Can you work these out from the model? Positions are in its coordinate system, mm. A direction names the side the tool comes from. Round coordinates to 2 decimals unless told otherwise and drop trailing zeros. Write each loop counter-clockwise with the first axis right and the second up, starting at its lowest first coordinate (ties: lowest second). Pieces come first, ordered by that corner, then holes. Notation, with made-up numbers: M -30,-7.75 L 16,-7.75 A36 ccw 16,29.25 Z; hole C -26,5.25 d10. An arc over 180 degrees is marked long. Use one line per item in the form item = value. Start each with the question number.
```python
from build123d import *

# Parameters (mm, degrees)
SKETCH1_R           = 113.19870133
BOSS_EXTRUDE1_DEPTH = 10
SKETCH3_R           = 10
BOSS_EXTRUDE2_DEPTH = 92
BOSS_EXTRUDE3_START = -10
SKETCH4_R           = 118.19870133
SKETCH4_R_2         = 113.19870133
BOSS_EXTRUDE3_DEPTH = 102
CUT_EXTRUDE1_START  = -59
CUT_EXTRUDE1_DEPTH  = 59


with BuildPart() as part:
    # Sketch1 → Boss-Extrude1 (new body)
    with BuildSketch(Plane(origin=(0, 0, 0), x_dir=(1, 0, 0), z_dir=(0, 1, 0))):
        with Locations(Location((0, 0, 0), (0, 0, 270))):
            Circle(SKETCH1_R)
    extrude(amount=BOSS_EXTRUDE1_DEPTH)

    # Sketch3 → Boss-Extrude2 (add)
    with BuildSketch(Plane(origin=(0, 10, 0), x_dir=(1, 0, 0), z_dir=(0, 1, 0))):
        with BuildLine():
            Line((11.81310243, 2.10964712), (146.802984355, 2.10964712))
            ThreePointArc((146.802984355, 2.10964712), (146.818142021, 0), (146.802984355, -2.10964712))
            Line((146.802984355, -2.10964712), (11.81310243, -2.10964712))
            ThreePointArc((11.81310243, -2.10964712), (10.811626415, -5.206604869), (9.014737429, -7.920511921))
            Line((9.014737429, -7.920511921), (93.179552163, -113.459851424))
            ThreePointArc((93.179552163, -113.459851424), (91.539614278, -114.78704563), (89.880775093, -116.090538354))
            Line((89.880775093, -116.090538354), (5.715960358, -10.55119885))
            ThreePointArc((5.715960358, -10.55119885), (2.670251207, -11.699134946), (-0.571908724, -11.986363936))
            Line((-0.571908724, -11.986363936), (-30.609983324, -143.591767687))
            ThreePointArc((-30.609983324, -143.591767687), (-32.670110084, -143.137104671), (-34.723491048, -142.652886392))
            Line((-34.723491048, -142.652886392), (-4.685416448, -11.047482641))
            ThreePointArc((-4.685416448, -11.047482641), (-7.481877622, -9.38197779), (-9.727895943, -7.02623943))
            Line((-9.727895943, -7.02623943), (-131.349577039, -65.596154143))
            ThreePointArc((-131.349577039, -65.596154143), (-132.278575204, -63.70200443), (-133.1802602, -61.794701388))
            Line((-133.1802602, -61.794701388), (-11.558579104, -3.224786676))
            ThreePointArc((-11.558579104, -3.224786676), (-12, 0), (-11.558579104, 3.224786676))
            Line((-11.558579104, 3.224786676), (-133.1802602, 61.794701388))
            ThreePointArc((-133.1802602, 61.794701388), (-132.278575204, 63.70200443), (-131.349577039, 65.596154143))
            Line((-131.349577039, 65.596154143), (-9.727895943, 7.02623943))
            ThreePointArc((-9.727895943, 7.02623943), (-7.481877622, 9.38197779), (-4.685416448, 11.047482641))
            Line((-4.685416448, 11.047482641), (-34.723491048, 142.652886392))
            ThreePointArc((-34.723491048, 142.652886392), (-32.670110084, 143.137104671), (-30.609983324, 143.591767687))
            Line((-30.609983324, 143.591767687), (-0.571908724, 11.986363936))
            ThreePointArc((-0.571908724, 11.986363936), (2.670251207, 11.699134946), (5.715960358, 10.55119885))
            Line((5.715960358, 10.55119885), (89.880775093, 116.090538354))
            ThreePointArc((89.880775093, 116.090538354), (91.539614278, 114.78704563), (93.179552163, 113.459851424))
            Line((93.179552163, 113.459851424), (9.014737429, 7.920511921))
            ThreePointArc((9.014737429, 7.920511921), (10.811626415, 5.206604869), (11.81310243, 2.10964712))
        make_face()
        with Locations(Location((0, 0, 0), (0, 0, 270))):
            Circle(SKETCH3_R, mode=Mode.SUBTRACT)
    extrude(amount=BOSS_EXTRUDE2_DEPTH)

    # Sketch4 → Boss-Extrude3 (add)
    with BuildSketch(Plane(origin=(0, 10, 0), x_dir=(1, 0, 0), z_dir=(0, 1, 0)).offset(BOSS_EXTRUDE3_START)):
        with Locations(Location((0, 0, 0), (0, 0, 270))):
            Circle(SKETCH4_R)
        Circle(SKETCH4_R_2, mode=Mode.SUBTRACT)
    extrude(amount=BOSS_EXTRUDE3_DEPTH)

    # Sketch5 → Cut-Extrude1 (cut)
    with BuildSketch(Plane(origin=(0, 10, 0), x_dir=(1, 0, 0), z_dir=(0, 1, 0)).offset(CUT_EXTRUDE1_START)):
        with BuildLine():
            Line((-113.173392965, 2.393555442), (-11.53804838, 2.393555442))
            ThreePointArc((-11.53804838, 2.393555442), (-10.204986578, 5.891851748), (-7.841904008, 8.795465286))
            Line((-7.841904008, 8.795465286), (-58.6595763, 96.814255619))
            ThreePointArc((-58.6595763, 96.814255619), (-98.032951027, 56.599350665), (-113.173392965, 2.393555442))
        make_face()
        with BuildLine():
            Line((-54.513816664, 99.207811061), (-3.696144372, 11.189020728))
            ThreePointArc((-3.696144372, 11.189020728), (0, 11.783703496), (3.696144372, 11.189020728))
            Line((3.696144372, 11.189020728), (54.513816664, 99.207811061))
            ThreePointArc((54.513816664, 99.207811061), (0, 113.19870133), (-54.513816664, 99.207811061))
        make_face()
        with BuildLine():
            Line((-58.6595763, -96.814255619), (-7.841904008, -8.795465286))
            ThreePointArc((-7.841904008, -8.795465286), (-10.204986578, -5.891851748), (-11.53804838, -2.393555442))
            Line((-11.53804838, -2.393555442), (-113.173392965, -2.393555442))
            ThreePointArc((-113.173392965, -2.393555442), (-98.032951027, -56.599350665), (-58.6595763, -96.814255619))
        make_face()
        with BuildLine():
            Line((54.513816664, -99.207811061), (3.696144372, -11.189020728))
            ThreePointArc((3.696144372, -11.189020728), (0, -11.783703496), (-3.696144372, -11.189020728))
            Line((-3.696144372, -11.189020728), (-54.513816664, -99.207811061))
            ThreePointArc((-54.513816664, -99.207811061), (0, -113.19870133), (54.513816664, -99.207811061))
        make_face()
        with BuildLine():
            Line((113.173392965, -2.393555442), (11.53804838, -2.393555442))
            ThreePointArc((11.53804838, -2.393555442), (10.204986578, -5.891851748), (7.841904008, -8.795465286))
            Line((7.841904008, -8.795465286), (58.6595763, -96.814255619))
            ThreePointArc((58.6595763, -96.814255619), (98.032951027, -56.599350665), (113.173392965, -2.393555442))
        make_face()
        with BuildLine():
            Line((58.6595763, 96.814255619), (7.841904008, 8.795465286))
            ThreePointArc((7.841904008, 8.795465286), (10.204986578, 5.891851748), (11.53804838, 2.393555442))
            Line((11.53804838, 2.393555442), (113.173392965, 2.393555442))
            ThreePointArc((113.173392965, 2.393555442), (98.032951027, 56.599350665), (58.6595763, 96.814255619))
        make_face()
    extrude(amount=CUT_EXTRUDE1_DEPTH, mode=Mode.SUBTRACT)


solid = part.part
```
1. Please list where these lines run through material, in increasing order: line 1 along X through (y, z) = (75, 0); line 2 along Z through (x, y) = (18, 8.5); line 3 along Z through (x, y) = (83, 60).
2. If we mould it in two halves opening along Z, with no side actions, what happens to faces 6 (the face through (83, 10, 104)), 7 (the face through (-27.38, 55.36, 129.44)), 8 (the face through (-56.583, 55.356, -24.907)), 9 (the face through (62, 5, -2.394))? For each: pulls with the +Z half, pulls with the -Z half, needs draft (parallel to the pull), parting line crosses it, or undercut.
3. If we section it at A-A (x = 32): State how many separate pieces and enclosed holes the cut face has, and give its area (3 significant figures).
4. If we section it at C-C (x = -95): List the corners of the cut face in (y, z) for me.
5. Will these pins go through, and if not, where does the flat tip stop? pin 1 (11.5 mm diameter, centred on x = -31.5, z = 122.5, fed in from -Y); pin 2 (8.5 mm diameter, centred on x = 131, y = 70, fed in from +Z); pin 3 (12 mm diameter, centred on y = 11.5, z = 95.5, fed in from -X).
6. Which directions (+Z, -Z, +X, -X, +Y, -Y) give clear straight access to the entire face, cutting with the end or side of a thin tool? Please do faces 1 (the face through (33.606, 4.93, -53.421)), 2 (the face through (-30, 10, 54)), 3 (the face through (-120.11, 55.36, -55.5)), 4 (the face through (-56.031, 55.356, -29.325)), 5 (the face through (-29, 10, 129)).
7. If we section it at B-B (z = -81): List the corners of the cut face in (x, y) for me.
Model answer:
q1.line_1 = -118.2 to -113.2, -12 to -10, 10 to 146.82
q1.line_2 = -116.82 to -111.76, -35.96 to -26.39, -2.39 to 2.39, 26.39 to 35.96, 111.76 to 116.82
q1.line_3 = -107.46 to -100.7, -84.15 to -76.97, -2.11 to 2.11, 76.97 to 84.15, 100.7 to 107.46
q2.face_6 = needs draft
q2.face_7 = pulls with the +Z half
q2.face_8 = undercut
q2.face_9 = undercut
q3.separate_pieces = 7
q3.enclosed_holes = 0
q3.area = 2,930 mm2
q4.outline = M 0,-70.33 L 102,-70.33 L 102,-61.55 L 0,-61.55 Z; M 0,-2.39 L 10,-2.39 L 10,2.39 L 0,2.39 Z; M 0,61.55 L 102,61.55 L 102,70.33 L 0,70.33 Z; M 10,-48.09 L 102,-48.09 L 102,-43.41 L 10,-43.41 Z; M 10,43.41 L 102,43.41 L 102,48.09 L 10,48.09 Z
q5.pin_1 = 10
q5.pin_2 = 2.11
q5.pin_3 = -77.21
q6.face_1 = -Y
q6.face_2 = +Y
q6.face_3 = -X, +Y, -Y
q6.face_4 = +Y, -Y
q6.face_5 = +Z, -X, -Y
q7.outline = M -86.08,0 L -79.08,0 L -79.08,102 L -86.08,102 Z; M -49.53,0 L -44,0 L -44,10 L -49.53,10 Z; M -20.65,10 L -16.32,10 L -16.32,102 L -20.65,102 Z; M 44,0 L 49.53,0 L 49.53,10 L 44,10 Z; M 61.9,10 L 67.29,10 L 67.29,102 L 61.9,102 Z; M 79.08,0 L 86.08,0 L 86.08,102 L 79.08,102 Z
